Source: three-view drawing plus pictorial views. Frame: mm from the lowest corner of the part. Round coordinates to 2 decimals unless told otherwise and drop trailing zeros. Loops run counter-clockwise (first coordinate to the right, second up) from the corner with the lowest first, then second, coordinate; pieces in that order, holes last. Notation, with made-up numbers: (-9, -8) -> (27, -8) arc R18 ccw to (27, 2) -> close; hole circle Ø11 at (38, 61). An arc over 180 degrees is marked (long way). One line per question, with ' | ' between items. Start each with the question number.
Q1. Contact query for flat-ended pins moving along their axis: P1, Ø1, axis at x = 33, y = 154, coming from the -Z side; P2, Ø4, axis at x = 22.86, y = 238.76, coming from the -Z side. Output: stop coordinate, or through.
Q2. Cut plane A-A on x = 153.67. Return loops of the section in (y, z) (3 decimals).
Q3. Material intervals for L1, parallel to X at y = 16.51, z = 1.5; L2, parallel to Y at x = 23, z = 1.85; L3, parallel to X at y = 198.12, z = 2.05, sorted ascending.
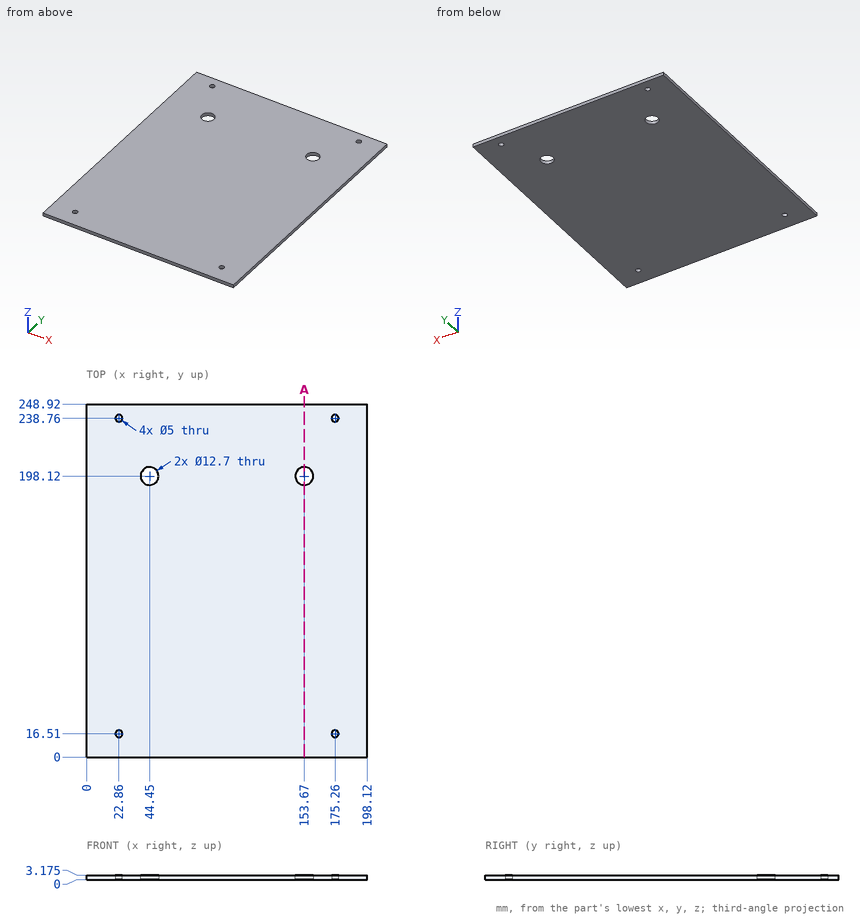
Results:
1) P1: z = 0 | P2: through
2) outline: (0, 0) -> (191.77, 0) -> (191.77, 3.175) -> (0, 3.175) -> close; (204.47, 0) -> (248.92, 0) -> (248.92, 3.175) -> (204.47, 3.175) -> close
3) L1: 0 to 20.36, 25.36 to 172.76, 177.76 to 198.12 | L2: 0 to 14.01, 19.01 to 236.26, 241.26 to 248.92 | L3: 0 to 38.1, 50.8 to 147.32, 160.02 to 198.12
